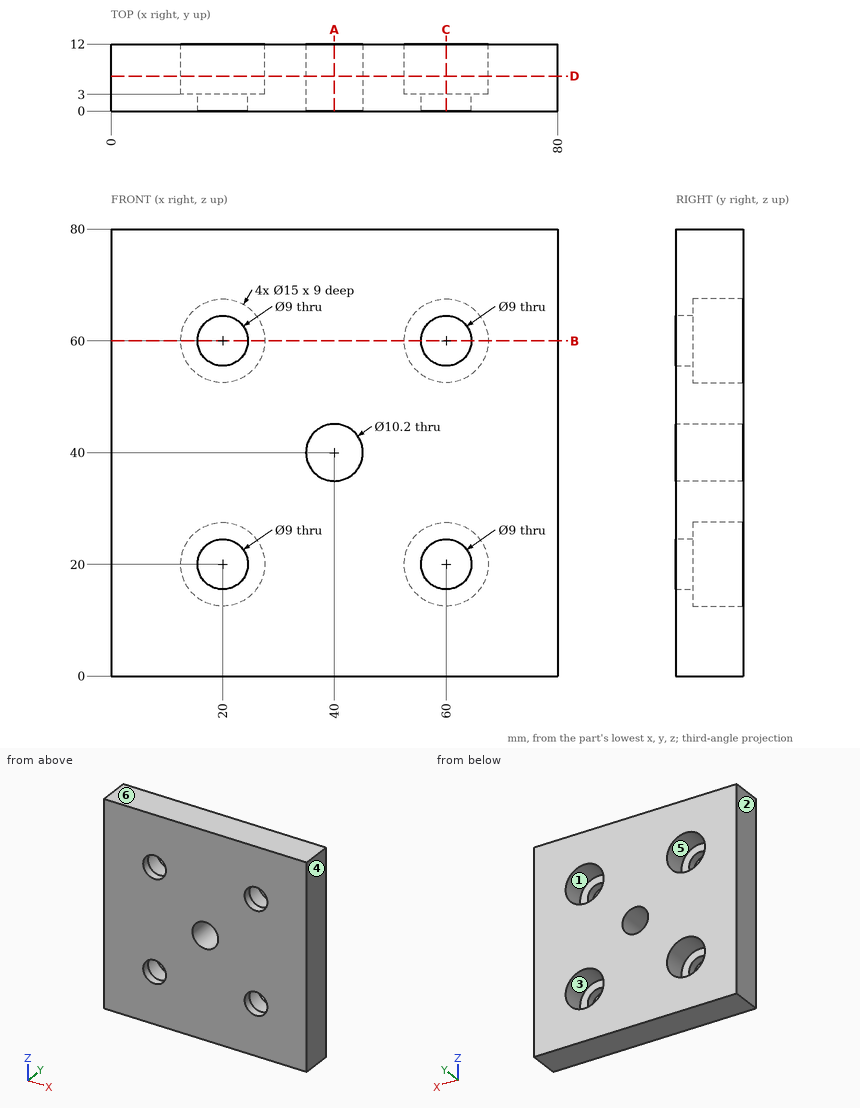
The figure shows three views and two pictorial views of one solid part (mm, origin at its lowest corner). Answer the questions. A direction names the side the tool comes from. Round coordinates to 2 decimals unless told otherwise and drop trailing zeros. Order: outer loops, then holes, each group sorted by start corner. A loop starts at its lowest first (then second) coordinate and runs counter-clockwise, first axis right, second up. Notation, with made-up numbers: M 3.5,87 L 36.5,87 A25 cw 36.5,104 Z; hole C 67,-4.5 d8. An arc over 180 degrees is marked long. Put each result on its own line as item: value. Start each with the question number.
Q1. Section D-D, the plane y = 6.25 is taken. Write down the section's boundary in (x, z).
Q2. A tool of negligible diameter and unlimited length cuts with its end or side. For the marked faces 1 and 2, from which of +Z, -Z, +X, -X, +Y, -Y can it reach the whole face along a straight path? Write none if from no direction.
Q3. Section C-C, the plane x = 60 is taken. Write down the section's boundary in (y, z), and give its area (3 significant figures).
Q4. Section B-B, the plane z = 60 is taken. Write down the section's boundary in (x, y).
Q5. Straight lines are drawn through the part: L1, parallel to X at y = 2, z = 60; L2, parallel to X at y = 7.5, z = 60. For each, find the intervals that lie inside material, in ascending order. Write a range as [from, to].
Q6. A flat-ended cylindrical pin translates along its axis: pin 1 (4.5 mm diameter, centred on x = 22.5, z = 21, fed in from +Y). Find the tip coordinate at first contact, or state that the pin passes through.
Q7. For a pull along X with two mould halves and no side action, classify the marked faces 3, 4, 5 and 6 as pulls with the +X half, pulls with the -X half, needs draft (parallel to the pull), parting line crosses it, or undercut.
Q8. Section A-A, the plane x = 40 is taken. Write down the section's boundary in (y, z).
Findings below:
1. outline: M 0,0 L 80,0 L 80,80 L 0,80 Z; hole C 20,20 d15; hole C 20,60 d15; hole C 40,40 d10.2; hole C 60,20 d15; hole C 60,60 d15
2. face 1: +Y
2. face 2: +Z, -Z, -X, +Y, -Y
3. outline: M 0,0 L 12,0 L 12,12.5 L 3,12.5 L 3,15.5 L 0,15.5 Z; M 0,24.5 L 3,24.5 L 3,27.5 L 12,27.5 L 12,52.5 L 3,52.5 L 3,55.5 L 0,55.5 Z; M 0,64.5 L 3,64.5 L 3,67.5 L 12,67.5 L 12,80 L 0,80 Z
3. area: 636 mm^2
4. outline: M 0,0 L 15.5,0 L 15.5,3 L 12.5,3 L 12.5,12 L 0,12 Z; M 24.5,0 L 55.5,0 L 55.5,3 L 52.5,3 L 52.5,12 L 27.5,12 L 27.5,3 L 24.5,3 Z; M 64.5,0 L 80,0 L 80,12 L 67.5,12 L 67.5,3 L 64.5,3 Z
5. L1: x = [0, 15.5], [24.5, 55.5], [64.5, 80]
5. L2: x = [0, 12.5], [27.5, 52.5], [67.5, 80]
6. pin 1: stops at y = 3
7. face 3: undercut
7. face 4: pulls with the +X half
7. face 5: undercut
7. face 6: needs draft
8. outline: M 0,0 L 12,0 L 12,34.9 L 0,34.9 Z; M 0,45.1 L 12,45.1 L 12,80 L 0,80 Z
